Build history of the part. All positions in model axes, mm. Round coordinates to 2 decimals unless told otherwise and drop trailing zeros. Write each loop counter-clockwise with the first axis right and the second up, starting at its lowest first coordinate (ties: lowest second). Pieces come first, ordered by that corner, then holes. Notation, with made-up numbers: (-25.5, -35) -> (30.5, -35) arc R18 ccw to (30.5, -17) -> close; hole circle Ø8 at (0, 44.5). An arc over 180 degrees is marked (long way). Answer as CSV lines item,"result".
Autodesk Inventor part; units mm, degrees
ref_plane "YZ Plane" through (0, 0, 0) normal (1, 0, 0) x (0, 1, 0)
ref_plane "XZ Plane" through (0, 0, 0) normal (0, 1, 0) x (-1, 0, 0)
ref_plane "XY Plane" through (0, 0, 0) normal (0, 0, 1) x (1, 0, 0)
sketch "Sketch1" plane through (0, 0, 0) normal (1, 0, 0) x (0, 1, 0)
  line L0 (0, 0) -> (21, 0)
  line L1 (0, 0) -> (0, 39)
  line L2 (0, 39) -> (2, 39)
  line L3 (2, 39) -> (2, 70)
  line L4 (2, 70) -> (18, 70)
  line L5 (18, 70) -> (18, 0)
  dimension "d0" = 78
  dimension "d2" = 18
  dimension "d3" = 140
  dimension "d6" = 2
revolve "Revolution1" add sketch "Sketch1" angle 360 about axis through (0, 0, 0) along (0, 1, 0)
sketch "Sketch2" plane through (0, 18, 0) normal (0, 1, 0) x (1, 0, 0)
  point P0 (0, 0)
  point P1 (-50, 0)
  point P2 (0, 50)
  point P3 (50, 0)
  point P4 (0, -50)
hole "Hole1" at (-50, 18, 0) at (0, 18, -50) at (50, 18, 0) at (0, 18, 50) direction (0, -1, 0) diameter 18 end through all
fillet "Fillet1" radius 2 1 edges at (0, 2, -39)
properties part number "vakkarima" material "Steel, Alloy"
1. Cut at D-D, the plane z = -50. Write the cut outline in (x, y), then the cut area to 3 significant figures.
Results found:
outline,"(-48.99, 2) -> (-9, 2) -> (-9, 18) -> (-48.99, 18) -> close; (9, 2) -> (48.99, 2) -> (48.99, 18) -> (9, 18) -> close"
area,"1,280 mm2"
2. Drop flat-ended pins along their axis: pin 1 Ø2 at (y, z) = (7.5, -34) entering from -X; pin 2 Ø10 at (x, y) = (-3.5, 12.5) entering from +Z; pin 3 Ø2 at (x, y) = (43, 16) entering from +Z; pin 4 Ø5 at (x, y) = (15, 8.5) entering from -Z. Give the stop position or say it passes through.
Results found:
pin 1,"stops at x = -61.73"
pin 2,"stops at z = 70"
pin 3,"stops at z = 56"
pin 4,"stops at z = -68.87"
3. Cut at A-A, the plane x = 0. Count the separate pieces of the cut face and the enclosed holes in it, then the cut area to 3 significant figures.
Results found:
separate pieces,"3"
enclosed holes,"0"
area,"1,820 mm2"
4. Cut at B-B, the plane y = 10.5. Write the cut outline in (x, z).
Results found:
outline,"circle Ø140 at (0, 0); hole circle Ø18 at (-50, 0); hole circle Ø18 at (0, -50); hole circle Ø18 at (0, 50); hole circle Ø18 at (50, 0)"
5. Mould opens along X. For faces 1 (the cylindrical face through (42.41, 9.89, 4.84)), 2 (the flat face through (-30, 2, 30)), 3 (the cylindrical face through (-42.594, 10.112, -55.55)) say: +X half, -X half, draft (parallel to the pull), parting line (faces both ways), or undercut.
Results found:
face 1,"undercut"
face 2,"draft"
face 3,"parting line"
6. Probe line 1 along X through (y, z) = (10.5, 0); line 2 along Z through (x, y) = (2, 12); line 3 along Z through (x, y) = (4, 12). List the from-to ranges inside material, lowest first.
Results found:
line 1,"x = -70 to -59, -41 to 41, 59 to 70"
line 2,"z = -69.97 to -58.77, -41.23 to 41.23, 58.77 to 69.97"
line 3,"z = -69.89 to -58.06, -41.94 to 41.94, 58.06 to 69.89"
7. Cut at C-C, the plane x = -50. Write the cut outline in (y, z), then the cut area to 3 significant figures.
Results found:
outline,"(2, -48.99) -> (18, -48.99) -> (18, -9) -> (2, -9) -> close; (2, 9) -> (18, 9) -> (18, 48.99) -> (2, 48.99) -> close"
area,"1,280 mm2"
